Autodesk Inventor part; units mm, degrees
ref_plane "YZ Plane" through (0, 0, 0) normal (1, 0, 0) x (0, 1, 0)
ref_plane "XZ Plane" through (0, 0, 0) normal (0, 1, 0) x (-1, 0, 0)
ref_plane "XY Plane" through (0, 0, 0) normal (0, 0, 1) x (1, 0, 0)
sketch "スケッチ1" plane through (0, 0, 0) normal (0, 0, 1) x (1, 0, 0)
  line L0 (50, -115) -> (-50, -115)
  line L1 (-50, -115) -> (-50, 115)
  line L2 (-50, 115) -> (50, 115)
  line L3 (50, 115) -> (50, -115)
  line L4 (50, -115) -> (-50, 115) construction
  line L5 (-50, -115) -> (50, 115) construction
  point P0 (0, 0)
  dimension "d0" = 230
  dimension "d1" = 100
extrude "押し出し1" add sketch "スケッチ1" along normal blind 3
sketch "スケッチ2" plane through (0, 0, 3) normal (0, 0, 1) x (1, 0, 0)
  line L0 (38, -105) -> (-38, -105)
  line L1 (-38, -105) -> (-38, 30)
  line L2 (-38, 30) -> (38, 30)
  line L3 (38, 30) -> (38, -105)
  line L4 (38, -105) -> (-38, 30) construction
  line L5 (-38, -105) -> (38, 30) construction
  line L6 (-50, -115) -> (50, -115)
  point P0 (0, 0)
  point P1 (0, -37.5)
  point P2 (0, -37.5)
  dimension "d4" = 76
  dimension "d5" = 135
  dimension "d6" = 10
hole "穴1" at (-38, -105, 3) at (38, -105, 3) at (38, 30, 3) at (-38, 30, 3) direction (0, 0, -1) diameter 3.2 end through all
sketch "スケッチ3" plane through (0, 0, 3) normal (0, 0, 1) x (1, 0, 0)
  line L0 (41, 60) -> (-41, 60)
  line L1 (-41, 60) -> (-41, 90)
  line L2 (-41, 90) -> (41, 90)
  line L3 (41, 90) -> (41, 60)
  line L4 (41, 60) -> (-41, 90) construction
  line L5 (-41, 60) -> (41, 90) construction
  circle A0 centre (-38, 30) radius 1.6
  point P0 (0, 0)
  point P1 (0, 75)
  dimension "d14" = 82
  dimension "d15" = 30
  dimension "d16" = 30
hole "穴2" at (-41, 60, 3) at (41, 60, 3) at (41, 90, 3) at (-41, 90, 3) direction (0, 0, -1) diameter 4.2 end through all
sketch "スケッチ4" plane through (0, 0, 3) normal (0, 0, 1) x (1, 0, 0)
  circle A0 centre (41, 90) radius 2.1
  circle A1 centre (-41, 60) radius 2.1
  circle A2 centre (41, 60) radius 2.1
  circle A3 centre (-41, 90) radius 2.1
  circle A4 centre (38, 30) radius 1.6
  circle A5 centre (-38, -105) radius 1.6
  circle A6 centre (38, -105) radius 1.6
  circle A7 centre (-38, 30) radius 1.6
  line L0 (50, 115) -> (-50, 115)
  line L1 (-50, 115) -> (-50, -115)
  line L2 (-50, -115) -> (50, -115)
  line L3 (50, -115) -> (50, 115)
  line L4 (-60, -125) -> (-60, 125)
  line L5 (-60, 125) -> (60, 125)
  line L6 (60, 125) -> (60, -125)
  line L7 (60, -125) -> (-60, -125)
  point P0 (0, 0)
  dimension "d24" = 10
extrude "押し出し2" add sketch "スケッチ4" against normal up to surface (3 mm away) contours L4 L5 L6 L7
sketch "スケッチ5" plane through (0, 0, 3) normal (0, 0, 1) x (1, 0, 0)
  line L0 (60, 125) -> (-60, 125)
  line L1 (-60, 125) -> (-60, -125)
  line L2 (-60, -125) -> (60, -125)
  line L3 (60, -125) -> (60, 125)
  circle A0 centre (41, 90) radius 2.1
  circle A1 centre (-41, 60) radius 2.1
  circle A2 centre (41, 60) radius 2.1
  circle A3 centre (-41, 90) radius 2.1
  circle A4 centre (38, 30) radius 1.6
  circle A5 centre (-38, -105) radius 1.6
  circle A6 centre (38, -105) radius 1.6
  circle A7 centre (-38, 30) radius 1.6
  line L4 (-55, -120) -> (-55, 120)
  line L5 (-55, 120) -> (55, 120)
  line L6 (55, 120) -> (55, -120)
  line L7 (55, -120) -> (-55, -120)
  point P0 (0, 0)
  point P1 (0, -120)
  point P2 (0, 120)
  point P3 (55, 0)
  point P4 (55, -60)
  point P5 (-55, -60)
  point P6 (-55, 60)
  point P7 (55, 60)
  point P8 (-55, 0)
  dimension "d27" = 5
  dimension "d28" = 60
  dimension "d29" = 60
hole "穴3" at (-55, -120, 3) at (55, -120, 3) at (0, -120, 3) at (0, 120, 3) at (-55, 120, 3) at (55, 120, 3) at (55, 0, 3) at (55, -60, 3) at (-55, -60, 3) at (-55, 60, 3) at (55, 60, 3) at (-55, 0, 3) direction (0, 0, -1) diameter 3.2 end through all
fillet "フィレット1" radius 2 4 edges at (-60, -125, 1.5) (60, -125, 1.5) (60, 125, 1.5) (-60, 125, 1.5)
sketch "スケッチ6" plane through (0, 0, 3) normal (0, 0, 1) x (1, 0, 0)
  circle A0 centre (55, 60) radius 1.6
  circle A1 centre (-55, -60) radius 1.6
  circle A2 centre (55, 0) radius 1.6
  circle A3 centre (-55, 120) radius 1.6
  circle A4 centre (0, -120) radius 1.6
  circle A5 centre (-55, -120) radius 1.6
  circle A6 centre (55, -120) radius 1.6
  circle A7 centre (0, 120) radius 1.6
  circle A8 centre (55, 120) radius 1.6
  circle A9 centre (55, -60) radius 1.6
  circle A10 centre (-55, 60) radius 1.6
  circle A11 centre (-55, 0) radius 1.6
  arc A12 (-58, 125) -> (-60, 123) centre (-58, 123) ccw
  line L0 (-60, 123) -> (-60, -123)
  arc A13 (-60, -123) -> (-58, -125) centre (-58, -123) ccw
  line L1 (-58, -125) -> (58, -125)
  arc A14 (58, -125) -> (60, -123) centre (58, -123) ccw
  line L2 (60, -123) -> (60, 123)
  arc A15 (60, 123) -> (58, 125) centre (58, 123) ccw
  line L3 (58, 125) -> (-58, 125)
  circle A16 centre (41, 90) radius 2.1
  circle A17 centre (-41, 60) radius 2.1
  circle A18 centre (41, 60) radius 2.1
  circle A19 centre (-41, 90) radius 2.1
  circle A20 centre (38, 30) radius 1.6
  circle A21 centre (-38, -105) radius 1.6
  circle A22 centre (38, -105) radius 1.6
  circle A23 centre (-38, 30) radius 1.6
  line L4 (22.5, 0) -> (7.5, 0) construction
  line L5 (22.5, 2.1) -> (7.5, 2.1)
  line L6 (7.5, -2.1) -> (22.5, -2.1)
  arc A24 (22.5, -2.1) -> (22.5, 2.1) centre (22.5, 0) ccw
  arc A25 (7.5, 2.1) -> (7.5, -2.1) centre (7.5, 0) ccw
  line L7 (22.5, -110) -> (7.5, -110) construction
  line L8 (22.5, -107.9) -> (7.5, -107.9)
  line L9 (7.5, -112.1) -> (22.5, -112.1)
  arc A26 (22.5, -112.1) -> (22.5, -107.9) centre (22.5, -110) ccw
  arc A27 (7.5, -107.9) -> (7.5, -112.1) centre (7.5, -110) ccw
  line L10 (22.5, 110) -> (7.5, 110) construction
  line L11 (22.5, 107.9) -> (7.5, 107.9)
  line L12 (7.5, 112.1) -> (22.5, 112.1)
  arc A28 (22.5, 107.9) -> (22.5, 112.1) centre (22.5, 110) ccw
  arc A29 (7.5, 112.1) -> (7.5, 107.9) centre (7.5, 110) ccw
  point P0 (15, 0)
  point P1 (15, -110)
  point P2 (15, 110)
  dimension "d38" = 4.2
  dimension "d39" = 4.2
  dimension "d40" = 4.2
  dimension "d41" = 110
  dimension "d42" = 110
  dimension "d43" = 15
  dimension "d46" = 45
extrude "押し出し3" cut sketch "スケッチ6" against normal blind 3 contours A24 L6 A25 L5 | A26 L9 A27 L8 | L11 A29 L12 A28
sketch "スケッチ7" plane through (0, 0, 3) normal (0, 0, 1) x (1, 0, 0)
  arc A0 (7.5, 112.1) -> (7.5, 107.9) centre (7.5, 110) ccw
  line L0 (7.5, 112.1) -> (22.5, 112.1)
  arc A1 (22.5, 107.9) -> (22.5, 112.1) centre (22.5, 110) ccw
  line L1 (22.5, 107.9) -> (7.5, 107.9)
  arc A2 (7.5, 2.1) -> (7.5, -2.1) centre (7.5, 0) ccw
  line L2 (7.5, 2.1) -> (22.5, 2.1)
  arc A3 (22.5, -2.1) -> (22.5, 2.1) centre (22.5, 0) ccw
  line L3 (22.5, -2.1) -> (7.5, -2.1)
  line L4 (22.5, -112.1) -> (7.5, -112.1)
  arc A4 (7.5, -107.9) -> (7.5, -112.1) centre (7.5, -110) ccw
  line L5 (7.5, -107.9) -> (22.5, -107.9)
  arc A5 (22.5, -112.1) -> (22.5, -107.9) centre (22.5, -110) ccw
  circle A6 centre (55, 60) radius 1.6
  circle A7 centre (-55, -60) radius 1.6
  circle A8 centre (55, 0) radius 1.6
  circle A9 centre (-55, 120) radius 1.6
  circle A10 centre (0, -120) radius 1.6
  circle A11 centre (-55, -120) radius 1.6
  circle A12 centre (55, -120) radius 1.6
  circle A13 centre (0, 120) radius 1.6
  circle A14 centre (55, 120) radius 1.6
  circle A15 centre (55, -60) radius 1.6
  circle A16 centre (-55, 60) radius 1.6
  circle A17 centre (-55, 0) radius 1.6
  arc A18 (-58, 125) -> (-60, 123) centre (-58, 123) ccw
  line L6 (-60, 123) -> (-60, -123)
  arc A19 (-60, -123) -> (-58, -125) centre (-58, -123) ccw
  line L7 (-58, -125) -> (58, -125)
  arc A20 (58, -125) -> (60, -123) centre (58, -123) ccw
  line L8 (60, -123) -> (60, 123)
  arc A21 (60, 123) -> (58, 125) centre (58, 123) ccw
  line L9 (58, 125) -> (-58, 125)
  circle A22 centre (41, 90) radius 2.1
  circle A23 centre (-41, 60) radius 2.1
  circle A24 centre (41, 60) radius 2.1
  circle A25 centre (-41, 90) radius 2.1
  circle A26 centre (38, 30) radius 1.6
  circle A27 centre (-38, -105) radius 1.6
  circle A28 centre (38, -105) radius 1.6
  circle A29 centre (-38, 30) radius 1.6
  point P0 (0, 0)
properties part number "Contorller_Mount"
Here's how the part is built. I have some questions about the finished solid (model axes, mm). Coordinates: 2 decimals unless noted, no trailing zeros. One line per question, with ' | ' between items.
(1) If we mould it in two halves opening along Y, with no side actions, what happens to faces 1 (the cylindrical face through (-39.722, 91.666, 1.479)), 2 (the flat face through (-1, 2, 0))? For each: pulls with the +Y half, pulls with the -Y half, needs draft (parallel to the pull), parting line crosses it, or undercut.
Report:
face 1: undercut | face 2: needs draft
(2) If I drill on L1, parallel to Y at x = 10, z = 0.2; L2, parallel to Y at x = -55, z = 1.35; L3, parallel to X at y = 60, z = 2.3, over which ranges is the centre line in solid material (lowest first)?
Report:
L1: y = -125 to -112.1, -107.9 to -2.1, 2.1 to 107.9, 112.1 to 125 | L2: y = -125 to -121.6, -118.4 to -61.6, -58.4 to -1.6, 1.6 to 58.4, 61.6 to 118.4, 121.6 to 125 | L3: x = -60 to -56.6, -53.4 to -43.1, -38.9 to 38.9, 43.1 to 53.4, 56.6 to 60
(3) Will these pins go through, and if not, where does the flat tip stop? pin 1 (3 mm diameter, centred on x = -23, y = 17.5, fed in from -Z); pin 2 (3 mm diameter, centred on x = -55, y = -120, fed in from +Z).
Report:
pin 1: stops at z = 0 | pin 2: passes through
